Could you check a few things on this model? Use its own coordinates, in mm. Face numbers are marked on the shaded views. A direction names the side the tool comes from. Coordinates: 2 decimals unless noted, no trailing zeros. Loops run counter-clockwise (first coordinate to the right, second up) from the corner with the lowest first, then second, coordinate; pieces in that order, holes last.
from build123d import *

# Parameters (mm, degrees)
SKETCH021_R           = 4.5
SKETCH021_R_2         = 1.5
PAD011_DEPTH          = 10
FILLET_R              = 4.5
SKETCH022_R           = 3
POCKET004_DEPTH       = 350.264033
POCKET004_DEPTH_BACK  = 350.264033
POLARPATTERN001_COUNT = 3
FILLET001_R           = 45
SKETCH025_R           = 1.5
POCKET005_DEPTH       = 304.699646
POLARPATTERN002_COUNT = 3


with BuildPart() as part:
    # Sketch021 → Pad011 (new body)
    with BuildSketch(Plane.XY):
        Polygon((-40.564433, -40.740341), (-55.564387, -14.759659), (-14.999954, 8.660227), (-14.999954, 55.5), (14.999954, 55.5), (14.999954, 8.660227), (55.564387, -14.759659), (40.564387, -40.740421), (0, -17.320455), align=None)
        Circle(SKETCH021_R, mode=Mode.SUBTRACT)
        with Locations((0, 17.320508)):
            Circle(SKETCH021_R_2, mode=Mode.SUBTRACT)
        with Locations((15, -8.660254)):
            Circle(SKETCH021_R_2, mode=Mode.SUBTRACT)
        with Locations((-15, -8.660254)):
            Circle(SKETCH021_R_2, mode=Mode.SUBTRACT)
    extrude(amount=PAD011_DEPTH)

    # Fillet
    fillet_edges = [part.edges().sort_by_distance(p)[0] for p in [
        (0, 55.5, 0),
        (48.064387, -27.75004, 0),
        (-48.06441, -27.75, 0),
        (48.064387, -27.75004, 10),
        (-48.06441, -27.75, 10),
        (0, 55.5, 10),
    ]]
    fillet(fillet_edges, radius=FILLET_R)

    # Sketch022 → Pocket004 (cut, two sides)
    with BuildSketch(Plane.YZ) as pocket004_sk:
        with Locations((50.5, 5)):
            Circle(SKETCH022_R)
    pocket004 = extrude(amount=-POCKET004_DEPTH, mode=Mode.SUBTRACT) + extrude(pocket004_sk.sketch, amount=POCKET004_DEPTH_BACK, mode=Mode.SUBTRACT)

    # PolarPattern001: Pocket004 ×3 about axis
    polarpattern001_axis = Axis((0, 0, 0), (0, 0, 1))
    for i in range(1, POLARPATTERN001_COUNT):
        add(pocket004.rotate(polarpattern001_axis, i * 360 / POLARPATTERN001_COUNT), mode=Mode.SUBTRACT)

    # Fillet001
    fillet001_edges = [part.edges().sort_by_distance(p)[0] for p in [
        (14.999954, 8.660227, 5),
        (-14.999954, 8.660227, 5),
        (0, -17.320455, 5),
    ]]
    fillet(fillet001_edges, radius=FILLET001_R)

    # Sketch025 (on Face5 of Fillet001) → Pocket005 (cut, through all)
    with BuildSketch(Plane.XY.offset(10)):
        with Locations((11.552559, 23.990381)):
            Circle(SKETCH025_R)
        with Locations((26.552559, -1.990381)):
            Circle(SKETCH025_R)
    pocket005 = extrude(amount=-POCKET005_DEPTH, mode=Mode.SUBTRACT)

    # PolarPattern002: Pocket005 ×3 about axis
    polarpattern002_axis = Axis((0, 0, 10), (0, 0, 1))
    for i in range(1, POLARPATTERN002_COUNT):
        add(pocket005.rotate(polarpattern002_axis, i * 360 / POLARPATTERN002_COUNT), mode=Mode.SUBTRACT)


solid = part.part
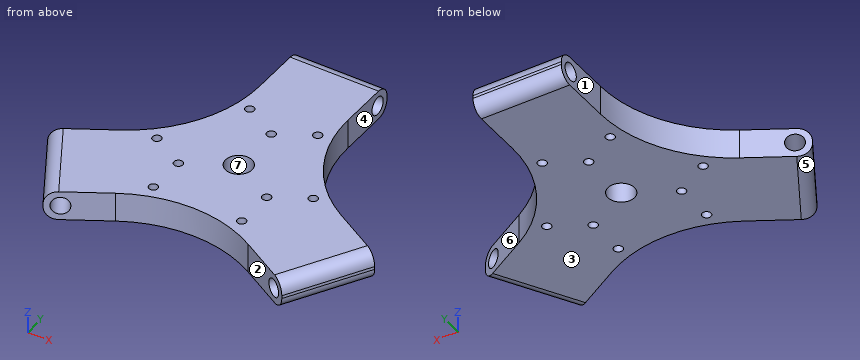
(1) For pin 1 (6 mm diameter, centred on y = 43.5, z = 7.5, fed in from +X); pin 2 (1 mm diameter, centred on y = -14, z = 1, fed in from -X); pin 3 (1.5 mm diameter, centred on y = -19.5, z = 8, fed in from +X), each with a flat end and sliding along its axis, tell me the tip position at first contact or that it passes through.
Answers:
pin 1: stops at x = 15
pin 2: stops at x = -54.55
pin 3: stops at x = 52.61
(2) I need wall thicknesses on probe 1 along Y at (x, z) = (-1.25, 5); probe 2 along X at (y, z) = (-9, 4.25); probe 3 along X at (y, z) = (-17, 4.5). Which ranges of each line are inside material? Lowest first, please.
Answers:
probe 1: y = -24.3 to -4.32, 4.32 to 16.49, 18.15 to 47.5, 53.5 to 55.5
probe 2: x = -45.59 to -16.46, -13.54 to 13.54, 16.46 to 45.59
probe 3: x = -54.27 to -51.91, -45.08 to 45.08, 51.91 to 54.27
(3) We'd pull the mould along X, two halves only. Please class the marked faces 5, 6 and 7: +X half, -X half, draft (parallel to the pull), parting line (faces both ways), or undercut.
Answers:
face 5: -X half
face 6: +X half
face 7: undercut
(4) Imagine slicing it at A-A, the plane x = 0. Write out the boundary of the cut face in (y, z).
Answers:
outline: (-24.28, 0) - (-4.5, 0) - (-4.5, 10) - (-24.28, 10) - close; (4.5, 0) - (15.82, 0) - (15.82, 10) - (4.5, 10) - close; (18.82, 0) - (51, 0) arc R4.5 ccw to (55.5, 4.5) - (55.5, 5.5) arc R4.5 ccw to (51, 10) - (18.82, 10) - close; hole circle Ø6 at (50.5, 5)
(5) Which directions (+Z, -Z, +X, -X, +Y, -Y) give clear straight access to the entire face, cutting with the end or side of a thin tool? Please do the marked faces 1, 2, 3 and 4.
Answers:
face 1: +Z, -Z, -X, +Y
face 2: +Z, -Z, -Y
face 3: -Z, +X, -X, +Y, -Y
face 4: +Z, -Z, +X, +Y
(6) Imagine slicing it at D-D, the plane x = -31. Write out the boundary of the cut face in (y, z), and give its area (4 significant figures).
Answers:
outline: (-35.22, 0) - (0.23, 0) - (0.23, 10) - (-35.22, 10) - close
area: 354.5 mm2
(7) Imagine slicing it at B-B, the plane z = 3.25. State how many separate pieces and enclosed holes the cut face has, and give its area (3 significant figures).
Answers:
separate pieces: 4
enclosed holes: 10
area: 4,350 mm2
